Autodesk Inventor part; units mm, degrees
ref_plane "YZ Plane" through (0, 0, 0) normal (1, 0, 0) x (0, 1, 0)
ref_plane "XZ Plane" through (0, 0, 0) normal (0, 1, 0) x (-1, 0, 0)
ref_plane "XY Plane" through (0, 0, 0) normal (0, 0, 1) x (1, 0, 0)
sketch "Sketch1" plane through (0, 0, 0) normal (0, 0, 1) x (1, 0, 0)
  circle A0 centre (0, 0) radius 4.445
  dimension "d0" = 8.89
extrude "Extrusion1" add sketch "Sketch1" along normal mid plane 50.8
sketch "Sketch2" plane through (0, 0, 25.4) normal (0, 0, 1) x (1, 0, 0)
  circle A0 centre (0, 0) radius 6.35
  dimension "d3" = 12.7
extrude "Extrusion2" add sketch "Sketch2" along normal blind 4.826
fillet "Fillet1" radius 3.302 1 edges at (-6.35, 0, 30.226)
mirror "Mirror1" about plane through (0, 0, 0) normal (0, 0, 1) of "Extrusion2", "Fillet1"
sketch "Sketch3" plane through (0, 0, 0) normal (1, 0, 0) x (0, 1, 0)
  line L0 (-9.525, -12.7) -> (9.525, -12.7)
  line L1 (9.525, -12.7) -> (9.525, 12.7)
  line L2 (9.525, 12.7) -> (-9.525, 12.7)
  line L3 (-9.525, 12.7) -> (-9.525, -12.7)
  line L4 (-9.525, -12.7) -> (9.525, 12.7) construction
  line L5 (9.525, -12.7) -> (-9.525, 12.7) construction
  point P0 (0, 0)
  dimension "d7" = 19.05
  dimension "d8" = 25.4
extrude "Extrusion3" add sketch "Sketch3" along normal mid plane 19.304
sketch "Sketch4" plane through (9.652, 0, 0) normal (1, 0, 0) x (0, 0, -1)
  point P0 (0, 0)
  point P1 (0, 0)
hole "Hole1" at (9.652, 0, 0) direction (-1, 0, 0) diameter 12.7 end through all
properties part number "Insert"
CAD build for the part. Positions are in the model's coordinates, mm. A direction names the side the tool comes from. Give positions to 0.01 mm unless a question says otherwise; leave off trailing zeros. Write each loop counter-clockwise with the first axis right and the second up, starting at its lowest first coordinate (ties: lowest second). Pieces come first, ordered by that corner, then holes. Notation, with made-up numbers: (58.5, 56) -> (78.5, 56) arc R28 ccw to (78.5, 80) -> close; hole circle Ø2 at (24, 0). An arc over 180 degrees is marked (long way). Write each question's results on one line, items separated by ' | '.
1. Cut at B-B, the plane x = -5.25. Give the number of separate pieces and of enclosed holes in the cut face, then the cut area to 3 significant figures.
Geometry check:
separate pieces: 3 | enclosed holes: 1 | area: 407 mm²
2. Which spindle directions (+Z, -Z, +X, -X, +Y, -Y) get a long thin tool onto all of the face, cutting with end or side? Do faces 5 (the flat face through (-2.3, 4.1, -12.7)), 6 (the cylindrical face through (-1.38, -6.2, -26.15)), 7 (the flat face through (-9.652, -6.5, 0.2)), 8 (the cylindrical face through (-1.38, 6.2, 26.15)), 9 (the flat face through (0, 9.525, 0)). Say none if no direction does.
Geometry check:
face 5: none | face 6: -Z | face 7: +Z, -Z, -X, +Y, -Y | face 8: +Z | face 9: +Z, -Z, +X, -X, +Y
3. Two-plate mould, pull along Z, no slides. Class faces 1 (the flat face through (0, 0, -30.226)), 2 (the flat face through (0, 0, 30.226)), 3 (the flat face through (9.652, -6.5, 0.2)), 4 (the cylindrical face through (-0.96, -4.34, -18.96)): pulls with the +Z half, pulls with the -Z half, needs draft (parallel to the pull), parting line crosses it, or undercut.
Geometry check:
face 1: pulls with the -Z half | face 2: pulls with the +Z half | face 3: needs draft | face 4: undercut
4. Cut at C-C, the plane y = -7.5. Write the cut outline in (x, z).
Geometry check:
outline: (-9.65, -12.7) -> (9.65, -12.7) -> (9.65, 12.7) -> (-9.65, 12.7) -> close
5. Drop flat-ended pins along their axis: P1, Ø1, axis at x = -5, z = 13.5, coming from the -Y side; P2, Ø2, axis at x = 4.5, z = 19, coming from the +Y side; P3, Ø10, axis at y = -6.5, z = 23.5, coming from the +X side; P4, Ø6, axis at x = -6.5, y = -0.5, coming from the -Z side. Give the stop position or say it passes through.
Geometry check:
P1: through | P2: y = 2.74 | P3: x = 6.07 | P4: z = -30.19
6. Cut at D-D, the plane z = 14. Write the cut outline in (x, y) (3 decimals), then the cut area to 3 significant figures.
Geometry check:
outline: circle Ø8.89 at (0, 0) | area: 62.1 mm²
7. Wall check: probe 1 along Y at (x, z) = (-2.5, 0) (3 decimals); probe 2 along Z at (x, y) = (-4, 4.25); probe 3 along Z at (x, y) = (5.75, 1.5). Give the ranges that are in metal, low to high. Write a range as [from, to].
Geometry check:
probe 1: [-9.525, -6.35], [6.35, 9.525] | probe 2: [-28.69, -25.4], [-12.7, -4.72], [4.72, 12.7], [25.4, 28.69] | probe 3: [-28.51, -25.4], [-12.7, -6.17], [6.17, 12.7], [25.4, 28.51]
8. Cut at A-A, the plane z = 0. Write the cut outline in (x, y) (3 decimals), then the cut area to 3 significant figures.
Geometry check:
outline: (-9.652, -9.525) -> (9.652, -9.525) -> (9.652, -6.35) -> (-9.652, -6.35) -> close; (-9.652, 6.35) -> (9.652, 6.35) -> (9.652, 9.525) -> (-9.652, 9.525) -> close | area: 123 mm²
